```python
from build123d import *

# Parameters (mm, degrees)
CROQUIS1_R              = 66
SALIENTE_EXTRUIR1_DEPTH = 80
CROQUIS2_R              = 39
SALIENTE_EXTRUIR2_DEPTH = 87
CROQUIS4_R              = 52.5
SALIENTE_EXTRUIR3_DEPTH = 138
SALIENTE_EXTRUIR4_DEPTH = 81.5
CROQUIS6_R              = 2.625
CORTAR_EXTRUIR1_DEPTH   = 81.5
SKETCH1_R               = 3.35
CUT_EXTRUDE1_DEPTH      = 8


with BuildPart() as part:
    # Croquis1 → Saliente-Extruir1 (new body)
    with BuildSketch(Plane.XY):
        Circle(CROQUIS1_R)
    extrude(amount=SALIENTE_EXTRUIR1_DEPTH)

    # Croquis2 → Saliente-Extruir2 (add)
    with BuildSketch(Plane.XY):
        Circle(CROQUIS2_R)
    extrude(amount=-SALIENTE_EXTRUIR2_DEPTH)

    # Croquis4 → Saliente-Extruir3 (add)
    with BuildSketch(Plane.XY.offset(-87)):
        Circle(CROQUIS4_R)
    extrude(amount=-SALIENTE_EXTRUIR3_DEPTH)

    # Croquis5 → Saliente-Extruir4 (add, symmetric)
    with BuildSketch(Plane(origin=(0, 0, 0), x_dir=(0, 0, -1), z_dir=(1, 0, 0))):
        Polygon((-77.192193157, 79.301093587), (-85.192193157, 79.301093587), (-85.192193157, -90.698906413), (239.707949332, -90.698906413), (239.707949332, -82.698906413), (-77.192193157, -82.698906413), align=None)
    extrude(amount=SALIENTE_EXTRUIR4_DEPTH, both=True)

    # Croquis6 → Cortar-Extruir1 (cut, symmetric)
    with BuildSketch(Plane.XY.offset(85.19)):
        with Locations((-55.9, 58.301093587)):
            Circle(CROQUIS6_R)
        with Locations((55.9, 58.301093587)):
            Circle(CROQUIS6_R)
        with Locations((55.9, -69.698906413)):
            Circle(CROQUIS6_R)
        with Locations((-55.9, -69.698906413)):
            Circle(CROQUIS6_R)
    extrude(amount=CORTAR_EXTRUIR1_DEPTH, both=True, mode=Mode.SUBTRACT)

    # Sketch1 → Cut-Extrude1 (cut)
    with BuildSketch(Plane(origin=(0, -82.698906413, 0), x_dir=(1, 0, 0), z_dir=(0, 1, 0))):
        with Locations((0, 151.628034649)):
            Circle(SKETCH1_R)
        with Locations((0, 171.628034649)):
            Circle(SKETCH1_R)
    extrude(amount=-CUT_EXTRUDE1_DEPTH, mode=Mode.SUBTRACT)


solid = part.part
```
Input: part model. Units: mm. Frame: model coordinates. A direction names the side the tool comes from. Give positions to 0.01 mm unless a question says otherwise; leave off trailing zeros. Loops run counter-clockwise (first coordinate to the right, second up) from the corner with the lowest first, then second, coordinate; pieces in that order, holes last. Notation, with made-up numbers: M -34,20 L 15,20 A11 cw 15,27 Z; hole C -10.5,79.5 d2. An arc over 180 degrees is marked long. Answer as CSV lines item,"result". Start each with the question number.
1. Reachability of faces 1 (the face through (-5.077, 38.668, -42.891)), 2 (the face through (37, -57, 77.192)), 3 (the face through (1, -82.699, -83)) from +Z, -Z, +X, -X, +Y, -Y: full face, straight path, thin tool, end or side. Return the list, or none.
2. Section C-C on y = 0. Return loops of the section in (x, z), plus the area to 3 significant figures.
3. Line query: L1, parallel to Z at x = 0, y = -86.5; L2, parallel to Y at x = 1, z = -124; L3, parallel to Z at x = -17, y = -38. Output: solid intervals per line, ascending.
4. Section A-A on x = 0. Return loops of the section in (y, z), plus the area to 3 significant figures.
5. Section B-B on z = -207. Return loops of the section in (x, y).
6. Pull-direction query (Z, two-part tool) for faces 4 (the face through (-1, 1, -225)), 5 (the face through (1, -90.699, -75)), 6 (the face through (-39, -4, -87)); classes: released by +Z, released by -Z, zero draft, split by the parting line, or undercut.
7. Section D-D on x = 69.5. Return loops of the section in (y, z), plus the area to 3 significant figures.
8. Pin query (flat end, axial travel): P1, Ø2, axis at y = 27.5, z = -133, coming from the +X side; P2, Ø5, axis at y = -9.5, z = -132.5, coming from the -X side; P3, Ø10, axis at y = 5, z = -34, coming from the -X side. Return the tip coordinate at first contact, or that it passes through.
Computed values:
1,face 1,"none"
1,face 2,"-Z"
1,face 3,"-Z, +X, -X"
2,outline,"M -81.5,77.19 L -66,77.19 L -66,0 L -39,0 L -39,-87 L -52.5,-87 L -52.5,-225 L 52.5,-225 L 52.5,-87 L 39,-87 L 39,0 L 66,0 L 66,77.19 L 81.5,77.19 L 81.5,85.19 L -81.5,85.19 Z"
2,area,"32,800 mm²"
3,L1,"z = -239.71 to -174.98, -168.28 to -154.98, -148.28 to 85.19"
3,L2,"y = -90.7 to -82.7, -52.49 to 52.49"
3,L3,"z = -225 to -87, 0 to 85.19"
4,outline,"M -90.7,-239.71 L -82.7,-239.71 L -82.7,-174.98 L -90.7,-174.98 Z; M -90.7,-168.28 L -82.7,-168.28 L -82.7,-154.98 L -90.7,-154.98 Z; M -90.7,-148.28 L -82.7,-148.28 L -82.7,77.19 L -66,77.19 L -66,0 L -39,0 L -39,-87 L -52.5,-87 L -52.5,-225 L 52.5,-225 L 52.5,-87 L 39,-87 L 39,0 L 66,0 L 66,77.19 L 79.3,77.19 L 79.3,85.19 L -90.7,85.19 Z"
4,area,"35,300 mm²"
5,outline,"M -81.5,-90.7 L 81.5,-90.7 L 81.5,-82.7 L -81.5,-82.7 Z; C 0,0 d105"
6,face 4,"released by -Z"
6,face 5,"zero draft"
6,face 6,"undercut"
7,outline,"M -90.7,-239.71 L -82.7,-239.71 L -82.7,77.19 L 79.3,77.19 L 79.3,85.19 L -90.7,85.19 Z"
7,area,"3,900 mm²"
8,P1,"stops at x = 45.32"
8,P2,"stops at x = -52.03"
8,P3,"stops at x = -39"
